Could you check a few things on this model? Use its own coordinates, in mm. A direction names the side the tool comes from. Give positions to 0.01 mm unless a question says otherwise; leave off trailing zeros. Write each loop counter-clockwise with the first axis right and the second up, starting at its lowest first coordinate (ties: lowest second). Pieces come first, ordered by that corner, then holes. Notation, with made-up numbers: (84, -21) - (121, -21) arc R14 cw to (121, -9) - close; hole circle Ø10 at (73.25, 63.5). An arc over 180 degrees is marked (long way). Answer as CSV lines item,"result". Start each with the question number.
Q1. If I drill on line 1 along X through (y, z) = (25, -34); line 2 along Z through (x, y) = (-8, 4.5); line 3 along Y through (x, z) = (27, -37), over which ranges is the centre line in solid material (lowest first)?
Q2. On a 3-axis mill with a long thin cutter (end or side, diameter ignored), from which of +Z, -Z, +X, -X, +Y, -Y can I reach the whole of each face in a straight line? I mean faces 1 (the face through (6, 19, -34)), 2 (the face through (-1, 10, 0)), 3 (the face through (42, 5, -38)), 4 (the face through (-21.4, 5.3, 25.2)), 5 (the face through (15, 4, -28)). Say none if no direction works.
Q3. We'd pull the mould along X, two halves only. Please class faces 6 (the face through (-29, 10, -26)), 7 (the face through (-27.5, 4, -3)), 8 (the face through (21.4, 5.4, 25.2)): pulls with the +X half, pulls with the -X half, needs draft (parallel to the pull), parting line crosses it, or undercut.
Q4. Imagine slicing it at A-A on x = 12. List the corners of the cut face in (y, z) for me, and give its area (3 significant figures).
Q5. Imagine slicing it at C-C on x = 24. List the corners of the cut face in (y, z) for me.
Q6. Will these pins go through, and if not, where does the flat tip stop? pin 1 Ø0.5 at (x, y) = (27, 28) entering from -Z; pin 2 Ø10 at (y, z) = (10, -29.5) entering from +X; pin 3 Ø14 at (x, z) = (-2.5, 16) entering from -Y; pin 4 Ø5 at (y, z) = (13.5, -18.5) entering from +X.
Q7. Imagine slicing it at B-B on z = -6. List the corners of the cut face in (x, y) for me, and give its area (3 significant figures).
Q8. Imagine slicing it at D-D on z = 17. List the corners of the cut face in (x, y) for me, and give its area (3 significant figures).
```python
from build123d import *

# Parameters (mm, degrees)
SKETCH_1_W                  = 110
SKETCH_1_H                  = 80
EXTRUDE_1_DEPTH             = 2
SKETCH_2_W                  = 58
SKETCH_2_H                  = 80
EXTRUDE_2_DEPTH             = 8
CUT_EXTRUDE_1_DEPTH         = 8
SKETCH_4_W                  = 58
SKETCH_4_H                  = 13
EXTRUDE_3_DEPTH             = 28
CHAMFER_1_SIZE              = 8
CHAMFER_1_SIZE2             = 4.618802154
CHAMFER_2_SIZE              = 5
CHAMFER_2_SIZE2             = 13.737387097
CHAMFER_3_SIZE              = 1
CHAMFER_3_SIZE2             = 5.67128182
EXTRUDE_5_REACH             = 28
EXTRUDE_5_DIRECTION_2_REACH = 86
SKETCH_5_W                  = 3.5
SKETCH_5_H                  = 8
CUT_EXTRUDE_2_DEPTH         = 31
SKETCH_6_W                  = 30
SKETCH_6_H                  = 20
CUT_EXTRUDE_3_DEPTH         = 9
SKETCH_7_W                  = 30
SKETCH_7_H                  = 3
EXTRUDE_4_DEPTH             = 4
SKETCH_8_W                  = 2.5
SKETCH_8_H                  = 3
CUT_EXTRUDE_4_DEPTH         = 0.2
SKETCH_10_R                 = 0.5
CUT_EXTRUDE_5_DEPTH         = 4
SKETCH_11_R                 = 0.5
CUT_EXTRUDE_6_DEPTH         = 4
CHAMFER_4_SIZE              = 3
CHAMFER_4_SIZE2             = 1.732050808
CHAMFER_5_SIZE              = 0.5
CHAMFER_5_SIZE2             = 0.288675135
CHAMFER_5_PART_2_SIZE       = 0.5
CHAMFER_5_PART_2_SIZE2      = 0.288675135
CHAMFER_5_PART_3_SIZE       = 0.5
CHAMFER_5_PART_3_SIZE2      = 0.288675135
CUT_EXTRUDE_7_DEPTH         = 8
SKETCH_14_W                 = 5
SKETCH_14_H                 = 10
CUT_EXTRUDE_8_DEPTH         = 3


with BuildPart() as part:
    # 草图1 → 凸台-拉伸1 (new body)
    with BuildSketch(Plane(origin=(0, 0, 0), x_dir=(1, 0, 0), z_dir=(0, 1, 0))):
        Rectangle(SKETCH_1_W, SKETCH_1_H)
    extrude(amount=EXTRUDE_1_DEPTH)

    # 草图2 → 凸台-拉伸2 (add)
    with BuildSketch(Plane(origin=(0, 2, 0), x_dir=(1, 0, 0), z_dir=(0, 1, 0))):
        Rectangle(SKETCH_2_W, SKETCH_2_H)
    extrude(amount=EXTRUDE_2_DEPTH)

    # 草图3 → 切除-拉伸1 (cut)
    with BuildSketch(Plane(origin=(0, 10, 0), x_dir=(1, 0, 0), z_dir=(0, 1, 0))):
        Polygon((-14, -40), (-29, -10), (-29, -40), align=None)
        Polygon((29, -40), (14, -40), (29, -10), align=None)
    extrude(amount=-CUT_EXTRUDE_1_DEPTH, mode=Mode.SUBTRACT)

    # 草图4 → 凸台-拉伸3 (add)
    with BuildSketch(Plane(origin=(0, 2, 0), x_dir=(1, 0, 0), z_dir=(0, 1, 0))):
        with Locations((0, 33.5)):
            Rectangle(SKETCH_4_W, SKETCH_4_H)
    extrude(amount=EXTRUDE_3_DEPTH)

    # 倒角1
    chamfer_1_edges = [part.edges().sort_by_distance(p)[0] for p in [
        (0, 30, -27),
    ]]
    chamfer_1_side = [part.faces().sort_by_distance(p)[0] for p in [
        (0, 20, -27),
    ]]
    chamfer(chamfer_1_edges, length=CHAMFER_1_SIZE, length2=CHAMFER_1_SIZE2, reference=chamfer_1_side[0])

    # 倒角2
    chamfer_2_edges = [part.edges().sort_by_distance(p)[0] for p in [
        (0, 10, 40),
    ]]
    chamfer_2_side = [part.faces().sort_by_distance(p)[0] for p in [
        (0, 3.522522523, 40),
    ]]
    chamfer(chamfer_2_edges, length=CHAMFER_2_SIZE, length2=CHAMFER_2_SIZE2, reference=chamfer_2_side[0])

    # 倒角3
    chamfer_3_edges = [part.edges().sort_by_distance(p)[0] for p in [
        (34.5, 2, 40),
        (-34.5, 2, 40),
    ]]
    chamfer_3_side = [part.faces().sort_by_distance(p)[0] for p in [
        (0, 1.690789474, 40),
    ]]
    chamfer(chamfer_3_edges, length=CHAMFER_3_SIZE, length2=CHAMFER_3_SIZE2, reference=chamfer_3_side[0])

    # 凸台-拉伸5: up to this face of the body (flat: up to its plane)
    extrude_5_end = Plane(part.part.faces().sort_by_distance((55, 0.987971654, -0.687592684))[0])
    # 草图12 → 凸台-拉伸5 (add, up to the picked face)
    with BuildSketch(Plane(origin=(29, 0, 0), x_dir=(0, 0, -1), z_dir=(1, 0, 0)), mode=Mode.PRIVATE) as extrude_5_sk1:
        Polygon((40, 2), (40, 7), (35, 2), align=None)
    extrude_5_tool1 = split(extrude(extrude_5_sk1.sketch, amount=EXTRUDE_5_REACH, mode=Mode.PRIVATE), bisect_by=extrude_5_end, keep=Keep.BOTH, mode=Mode.PRIVATE)
    add(extrude_5_tool1.solids().sort_by_distance((29, 3.666667, -38.333333))[0])

    # 凸台-拉伸5 direction 2: up to this face of the body (flat: up to its plane)
    extrude_5_direction_2_end = Plane(part.part.faces().sort_by_distance((-55, 0.987971654, -0.687592684))[0])
    # 草图12 → 凸台-拉伸5 direction 2 (add, up to the picked face)
    with BuildSketch(Plane(origin=(29, 0, 0), x_dir=(0, 0, -1), z_dir=(1, 0, 0)), mode=Mode.PRIVATE) as extrude_5_direction_2_sk1:
        Polygon((40, 2), (40, 7), (35, 2), align=None)
    extrude_5_direction_2_tool1 = split(extrude(extrude_5_direction_2_sk1.sketch, amount=-EXTRUDE_5_DIRECTION_2_REACH, mode=Mode.PRIVATE), bisect_by=extrude_5_direction_2_end, keep=Keep.BOTH, mode=Mode.PRIVATE)
    add(extrude_5_direction_2_tool1.solids().sort_by_distance((29, 3.666667, -38.333333))[0])

    # 草图5 → 切除-拉伸2 (cut, through all)
    with BuildSketch(Plane.XZ):
        with Locations((-4.25, -34)):
            Rectangle(SKETCH_5_W, SKETCH_5_H)
        with Locations((4.25, -34)):
            Rectangle(SKETCH_5_W, SKETCH_5_H)
    extrude(amount=-CUT_EXTRUDE_2_DEPTH, mode=Mode.SUBTRACT)

    # 草图6 → 切除-拉伸3 (cut)
    with BuildSketch(Plane.XZ):
        with Locations((0, -28)):
            Rectangle(SKETCH_6_W, SKETCH_6_H)
    extrude(amount=-CUT_EXTRUDE_3_DEPTH, mode=Mode.SUBTRACT)

    # 草图7 → 凸台-拉伸4 (add)
    with BuildSketch(Plane.XZ.offset(-9)):
        with Locations((0, -27.5)):
            Rectangle(SKETCH_7_W, SKETCH_7_H)
    extrude(amount=EXTRUDE_4_DEPTH)

    # 草图8 → 切除-拉伸4 (cut)
    with BuildSketch(Plane.XZ.offset(-5)):
        with Locations((-4.25, -27.5)):
            Rectangle(SKETCH_8_W, SKETCH_8_H)
        with Locations((4.25, -27.5)):
            Rectangle(SKETCH_8_W, SKETCH_8_H)
    extrude(amount=-CUT_EXTRUDE_4_DEPTH, mode=Mode.SUBTRACT)

    # 草图10 → 切除-拉伸5 (cut)
    with BuildSketch(Plane.XZ.offset(-5)):
        with Locations((-8, -27.5)):
            Circle(SKETCH_10_R)
        with Locations((8, -27.5)):
            Circle(SKETCH_10_R)
        with Locations((0, -27.5)):
            Circle(SKETCH_10_R)
    extrude(amount=-CUT_EXTRUDE_5_DEPTH, mode=Mode.SUBTRACT)

    # 草图11 → 切除-拉伸6 (cut)
    with BuildSketch(Plane(origin=(0, 0, -40), x_dir=(-1, 0, 0), z_dir=(0, 0, -1))):
        with Locations((-52.5, 2)):
            Circle(SKETCH_11_R)
        with Locations((52.5, 2)):
            Circle(SKETCH_11_R)
        with Locations((-27, 28)):
            Circle(SKETCH_11_R)
        with Locations((27, 28)):
            Circle(SKETCH_11_R)
    extrude(amount=-CUT_EXTRUDE_6_DEPTH, mode=Mode.SUBTRACT)

    # 倒角4
    chamfer_4_edges = [part.edges().sort_by_distance(p)[0] for p in [
        (0, 10, -27),
    ]]
    chamfer_4_side = [part.faces().sort_by_distance(p)[0] for p in [
        (0, 16, -27),
    ]]
    chamfer(chamfer_4_edges, length=CHAMFER_4_SIZE, length2=CHAMFER_4_SIZE2, reference=chamfer_4_side[0])

    # 倒角5
    chamfer_5_edges = [part.edges().sort_by_distance(p)[0] for p in [
        (29, 10, -7.633974596),
        (24.934346774, 10, 18.131306451),
    ]]
    chamfer_5_side = [part.faces().sort_by_distance(p)[0] for p in [
        (0, 10, -0.444462332),
    ]]
    chamfer(chamfer_5_edges, length=CHAMFER_5_SIZE, length2=CHAMFER_5_SIZE2, reference=chamfer_5_side[0])

    # 倒角5 part 2
    chamfer_5_part_2_edges = [part.edges().sort_by_distance(p)[0] for p in [
        (-29, 10, -7.633974596),
    ]]
    chamfer_5_part_2_side = [part.faces().sort_by_distance(p)[0] for p in [
        (-29, 17.5, -27.573061951),
    ]]
    chamfer(chamfer_5_part_2_edges, length=CHAMFER_5_PART_2_SIZE, length2=CHAMFER_5_PART_2_SIZE2, reference=chamfer_5_part_2_side[0])

    # 倒角5 part 3
    chamfer_5_part_3_edges = [part.edges().sort_by_distance(p)[0] for p in [
        (-24.934346774, 10, 18.131306451),
    ]]
    chamfer_5_part_3_side = [part.faces().sort_by_distance(p)[0] for p in [
        (-22.269129124, 5.556709809, 23.461741751),
    ]]
    chamfer(chamfer_5_part_3_edges, length=CHAMFER_5_PART_3_SIZE, length2=CHAMFER_5_PART_3_SIZE2, reference=chamfer_5_part_3_side[0])

    # 草图13 → 切除-拉伸7 (cut)
    with BuildSketch(Plane.XZ):
        Polygon((27.5, -16), (-27.5, -16), (-27.5, 9.67128182), (-14.5, 30), (14.5, 30), (27.5, 9.67128182), align=None)
    extrude(amount=-CUT_EXTRUDE_7_DEPTH, mode=Mode.SUBTRACT)

    # 草图14 → 切除-拉伸8 (cut)
    with BuildSketch(Plane(origin=(0, 0, -40), x_dir=(-1, 0, 0), z_dir=(0, 0, -1))):
        Rectangle(SKETCH_14_W, SKETCH_14_H)
    extrude(amount=-CUT_EXTRUDE_8_DEPTH, mode=Mode.SUBTRACT)


solid = part.part
```
Conclusion:
1,line 1,"-29 to -6, -2.5 to 2.5, 6 to 29"
1,line 2,"-40 to -38, -18 to -16, 30 to 40"
1,line 3,"0 to 27.5, 28.5 to 30"
2,face 1,"+Y, -Y"
2,face 2,"+Z, +X, -X, +Y"
2,face 3,"+Z, +X, +Y"
2,face 4,"+Z, -X, +Y"
2,face 5,"-Y"
3,face 6,"pulls with the -X half"
3,face 7,"undercut"
3,face 8,"pulls with the +X half"
4,outline,"(0, -40) - (30, -40) - (30, -31.62) - (22, -27) - (13, -27) - (10, -25.27) - (10, 26.26) - (5, 40) - (0, 40) - (0, 30) - (8, 30) - (8, -16) - (0, -16) - (0, -18) - (9, -18) - (9, -26) - (5, -26) - (5, -29) - (9, -29) - (9, -38) - (0, -38) - close"
4,area,"474 mm^2"
5,outline,"(0, -40) - (30, -40) - (30, -31.62) - (22, -27) - (13, -27) - (10, -25.27) - (10, 18.88) - (9.71, 20) - (2, 20) - (2, 34.33) - (1, 40) - (0, 40) - (0, 15.14) - (8, 15.14) - (8, -16) - (0, -16) - close"
6,pin 1,"z = -36"
6,pin 2,"x = 29"
6,pin 3,"y = 8"
6,pin 4,"through"
7,outline,"(-55, 0) - (-27.5, 0) - (-27.5, 8) - (27.5, 8) - (27.5, 0) - (55, 0) - (55, 2) - (29, 2) - (29, 9.71) - (28.5, 10) - (-28.71, 10) - (-29, 9.5) - (-29, 2) - (-55, 2) - close"
7,area,"244 mm^2"
8,outline,"(-55, 0) - (-22.81, 0) - (-22.81, 8) - (22.81, 8) - (22.81, 0) - (55, 0) - (55, 2) - (25.5, 2) - (25.5, 9.71) - (24.94, 10) - (-25.18, 10) - (-25.5, 9.5) - (-25.5, 2) - (-55, 2) - close"
8,area,"263 mm^2"
